from build123d import *

# Parameters (mm, degrees)
F0_R     = 1.5
F1_DEPTH = 3.2


with BuildPart() as f1:
    # F0 (on Top) → F1 (new body)
    with BuildSketch(Plane.XY):
        Polygon((26.8, 25), (26.8, 30), (-26.8, 30), (-26.8, 25), (-30, 25), (-30, 20), (-26.8, 20), (-26.8, 15), (-30, 15), (-30, 10), (-26.8, 10), (-26.8, 5), (-30, 5), (-30, 0), (-26.8, 0), (-26.8, -5), (-30, -5), (-30, -10), (-26.8, -10), (-26.8, -15), (-30, -15), (-30, -20), (-26.8, -20), (-26.8, -25), (-30, -25), (-30, -30), (30, -30), (30, -25), (26.8, -25), (26.8, -20), (30, -20), (30, -15), (26.8, -15), (26.8, -10), (30, -10), (30, -5), (26.8, -5), (26.8, 0), (30, 0), (30, 5), (26.8, 5), (26.8, 10), (30, 10), (30, 15), (26.8, 15), (26.8, 20), (30, 20), (30, 25), align=None)
        with Locations((0, -21.5)):
            Circle(F0_R, mode=Mode.SUBTRACT)
        with Locations((-21.5, 0)):
            Circle(F0_R, mode=Mode.SUBTRACT)
        with Locations((21.5, 0)):
            Circle(F0_R, mode=Mode.SUBTRACT)
        with Locations((0, 21.5)):
            Circle(F0_R, mode=Mode.SUBTRACT)
    extrude(amount=F1_DEPTH)


solid = f1.part
The listing builds one solid part. Answer for the finished solid, in the listing's coordinates (mm). A direction names the side the tool comes from. Give positions to 0.01 mm unless a question says otherwise; leave off trailing zeros. Order: outer loops, then holes, each group sorted by start corner. A loop starts at its lowest first (then second) coordinate and runs counter-clockwise, first axis right, second up. Notation, with made-up numbers: (27.5, -33) -> (49.5, -33) arc R25 ccw to (49.5, -10) -> close; hole circle Ø8 at (83.5, 58). An arc over 180 degrees is marked (long way). Put each result on its own line as item: value.
Item 1: For faces 1 (the face through (28, -5, 2)), 2 (the face through (-26.8, 28, 2)), 3 (the face through (-26.8, 8, 2)), 4 (the face through (20, 0, 2)), determine the directions among +Z, -Z, +X, -X, +Y, -Y from which every point of the face is accessible in a straight line to the end or side of a thin tool.
Established:
face 1: +Z, -Z, +X
face 2: +Z, -Z, -X, +Y
face 3: +Z, -Z, -X
face 4: +Z, -Z
Item 2: A cutting plane is placed at B-B on x = 21.5. Give the vertices of the cut face in (y, z), plus the area to 3 significant figures.
Established:
outline: (-30, 0) -> (-1.5, 0) -> (-1.5, 3.2) -> (-30, 3.2) -> close; (1.5, 0) -> (30, 0) -> (30, 3.2) -> (1.5, 3.2) -> close
area: 182 mm^2
Item 3: Given P1, Ø1, axis at x = 28, z = 2, coming from the +Y side; P2, Ø1.6, axis at y = 7, z = 1.5, coming from the -X side; P3, Ø1.5, axis at y = -21, z = 1.5, coming from the +X side, each flat-ended and moving along its own axis, determine where each tip first touches the part or whether it passes through.
Established:
P1: stops at y = 25
P2: stops at x = -26.8
P3: stops at x = 26.8
Item 4: Straight lines are drawn through the part: line 1 (Y direction, x = 0, z = 0.85); line 2 (Y direction, x = 21.5, z = 2.05); line 3 (X direction, y = -2, z = 2.85). For each, find the intervals that lie inside material, in ascending order.
Established:
line 1: y = -30 to -23, -20 to 20, 23 to 30
line 2: y = -30 to -1.5, 1.5 to 30
line 3: x = -26.8 to 26.8
Item 5: For a pull along Y with two mould halves and no side action, classify faces 5 (the face through (26.8, 17, 2)), 6 (the face through (30, -18, 2)), 7 (the face through (28, -10, 2)) as released by +Y, released by -Y, zero draft, split by the parting line, or undercut.
Established:
face 5: undercut
face 6: zero draft
face 7: undercut
Item 6: A cutting plane is placed at D-D on z = 2.7. Count the separate pieces of the cut face and the enclosed holes in it, plus the area to 3 significant figures.
Established:
separate pieces: 1
enclosed holes: 4
area: 3,380 mm^2
Item 7: A cutting plane is placed at A-A on x = 0. Give the vertices of the cut face in (y, z).
Established:
outline: (-30, 0) -> (-23, 0) -> (-23, 3.2) -> (-30, 3.2) -> close; (-20, 0) -> (20, 0) -> (20, 3.2) -> (-20, 3.2) -> close; (23, 0) -> (30, 0) -> (30, 3.2) -> (23, 3.2) -> close
